Source: CAD feature listing. Evaluate the final solid. Frame: model axes, mm. A direction names the side the tool comes from. Coordinates: 2 decimals unless noted, no trailing zeros. Loops run counter-clockwise (first coordinate to the right, second up) from the corner with the lowest first, then second, coordinate; pieces in that order, holes last.
from build123d import *

# Parameters (mm, degrees)
F0_W     = 254
F0_H     = 203.2
F0_R     = 3.175
F0_R_2   = 1.778
F1_DEPTH = 6.35
F2_SIZE  = 0.508
F3_SIZE  = 2.54


with BuildPart() as f1:
    # F0 (on Top) → F1 (new body)
    with BuildSketch(Plane.XY):
        with Locations((14.533197, 0)):
            Rectangle(F0_W, F0_H)
        with Locations((-99.898785, -88.9)):
            Circle(F0_R, mode=Mode.SUBTRACT)
        with BuildLine():
            ThreePointArc((27.233197, -69.322012), (8.183197, -88.372012), (-10.866803, -69.322012))
            Line((-10.866803, -69.322012), (-10.866803, 32.277988))
            ThreePointArc((-10.866803, 32.277988), (8.183197, 51.327988), (27.233197, 32.277988))
            Line((27.233197, 32.277988), (27.233197, -69.322012))
        make_face(mode=Mode.SUBTRACT)
        with Locations((128.833197, -88.9)):
            Circle(F0_R, mode=Mode.SUBTRACT)
        with Locations((-93.416854, 12.7)):
            Circle(F0_R_2, mode=Mode.SUBTRACT)
        with Locations((-93.416854, 50.8)):
            Circle(F0_R_2, mode=Mode.SUBTRACT)
        with Locations((-26.741854, 12.7)):
            Circle(F0_R_2, mode=Mode.SUBTRACT)
        with Locations((-26.741854, 50.8)):
            Circle(F0_R_2, mode=Mode.SUBTRACT)
        with Locations((-99.766803, 88.9)):
            Circle(F0_R, mode=Mode.SUBTRACT)
        with Locations((128.833197, 88.9)):
            Circle(F0_R, mode=Mode.SUBTRACT)
    extrude(amount=F1_DEPTH)

    # F2
    f2_edges = [f1.edges().sort_by_distance(p)[0] for p in [
        (141.533197, 0, 6.35),
        (14.533197, -101.6, 6.35),
        (14.533197, 101.6, 6.35),
        (-112.466803, 0, 6.35),
        (-112.466803, 0, 0),
        (14.533197, -101.6, 0),
        (141.533197, 0, 0),
        (14.533197, 101.6, 0),
        (-10.866803, -18.522012, 0),
        (-10.866803, -18.522012, 6.35),
        (-103.073785, -88.9, 0),
        (125.658197, -88.9, 0),
        (125.658197, 88.9, 0),
        (-102.941803, 88.9, 0),
    ]]
    chamfer(f2_edges, length=F2_SIZE)

    # F3
    f3_edges = [f1.edges().sort_by_distance(p)[0] for p in [
        (-102.941803, 88.9, 6.35),
        (-103.073785, -88.9, 6.35),
        (125.658197, 88.9, 6.35),
        (125.658197, -88.9, 6.35),
        (-95.194854, 12.7, 0),
        (-28.519854, 12.7, 0),
        (-28.519854, 50.8, 0),
        (-95.194854, 50.8, 0),
    ]]
    chamfer(f3_edges, length=F3_SIZE)


solid = f1.part
Q1. Line query: line 1 along X through (y, z) = (28, 0.5); line 2 along X through (y, z) = (91, 1.75); line 3 along Y through (x, z) = (130.5, 6.25). Output: solid intervals per line, ascending.
Q2. Draft query along Y for faces 1 (the cylindrical face through (8.602, -88.367, 3.138)), 2 (the flat face through (-112.467, -1, 3)), 3 (the flat face through (13, 101.6, 3)). Return one class per face: +Y half, -Y half, draft (parallel to the pull), parting line (faces both ways), or undercut.
Q3. Section B-B, the plane y = -28.5. Return the cut outline in (x, z), plus the area to 3 significant figures.
Q4. Access query for faces 4 (the conical face through (8.605, -88.512, 0.363)), 5 (the flat face through (-15, 1, 6.35)), 6 (the conical face through (7.76, 51.47, 5.99)). Directions: +Z, -Z, +X, -X, +Y, -Y. A direction counts if a zero-diameter tool reaches every point of the face in a straight line with its end or side. Return the directions, or none.
Q5. Section A-A, the plane y = 88.9. Return the cut outline in (x, z), plus the area to 3 significant figures.
Q6. Contact query for flat-ended pins moving along their axis: pin 1 Ø10 at (x, y) = (-99.9, -88.9) entering from +Z; pin 2 Ø8.5 at (x, y) = (128.83, -88.9) entering from +Z; pin 3 Ø5.5 at (x, y) = (128.83, 88.9) entering from -Z; pin 4 Ø4.5 at (x, y) = (-93.42, 50.8) entering from -Z. Output: stop coordinate, or through.
Derived:
1. line 1: x = -112.46 to -10.87, 27.24 to 141.53
1. line 2: x = -112.47 to -102.15, -97.39 to 126.45, 131.21 to 141.53
1. line 3: y = -101.19 to -94.26, -83.54 to 83.54, 94.26 to 101.19
2. face 1: undercut
2. face 2: draft
2. face 3: +Y half
3. outline: (-112.47, 0.51) - (-111.96, 0) - (-11.37, 0) - (-10.87, 0.51) - (-10.87, 5.84) - (-11.37, 6.35) - (-111.96, 6.35) - (-112.47, 5.84) - close; (27.23, 0.51) - (27.74, 0) - (141.03, 0) - (141.53, 0.51) - (141.53, 5.84) - (141.03, 6.35) - (27.74, 6.35) - (27.23, 5.84) - close
3. area: 1,370 mm2
4. face 4: -Z
4. face 5: +Z, +X, -X, +Y, -Y
4. face 6: +Z
5. outline: (-112.47, 0.51) - (-111.96, 0) - (-103.45, 0) - (-102.94, 0.51) - (-102.94, 3.81) - (-105.48, 6.35) - (-111.96, 6.35) - (-112.47, 5.84) - close; (-96.59, 0.51) - (-96.08, 0) - (125.15, 0) - (125.66, 0.51) - (125.66, 3.81) - (123.12, 6.35) - (-94.05, 6.35) - (-96.59, 3.81) - close; (132.01, 0.51) - (132.52, 0) - (141.03, 0) - (141.53, 0.51) - (141.53, 5.84) - (141.03, 6.35) - (134.55, 6.35) - (132.01, 3.81) - close
5. area: 1,520 mm2
6. pin 1: stops at z = 5.64
6. pin 2: stops at z = 4.89
6. pin 3: passes through
6. pin 4: stops at z = 2.06
